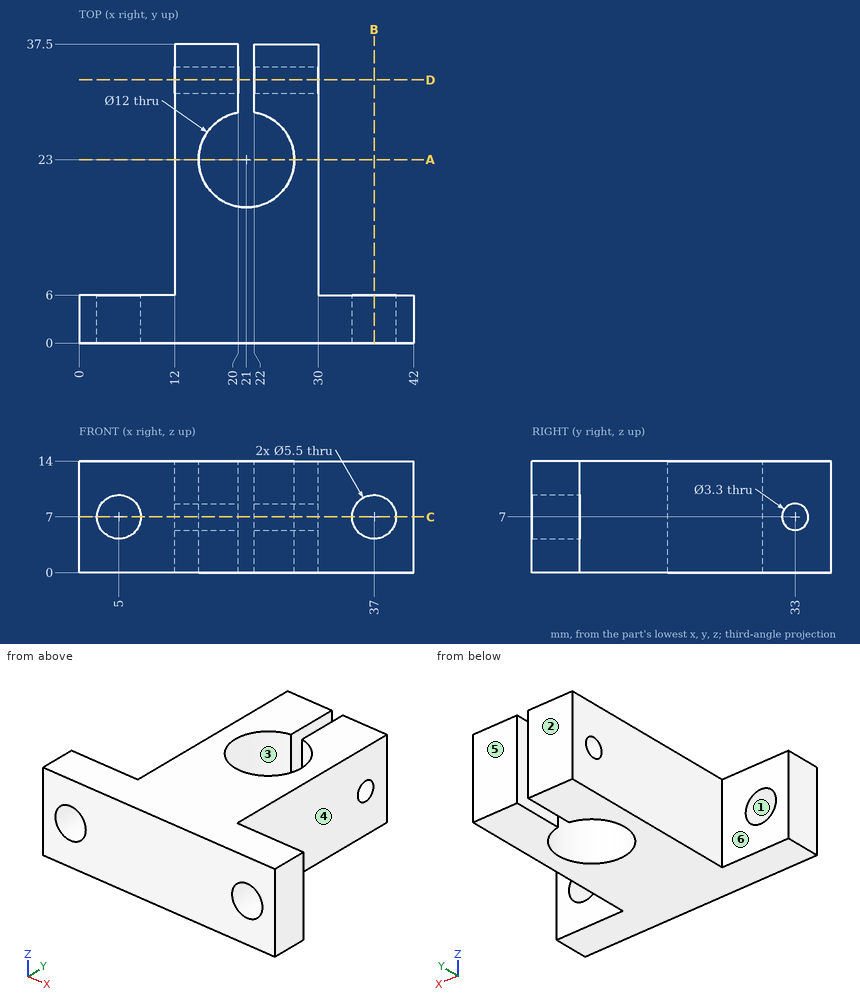
Study the drawing (mm; zero at the part's minimum x, y, z) and answer. A direction names the side the tool comes from. Give positions to 0.01 mm unless a question says otherwise; leave off trailing zeros. Write each loop counter-clockwise with the first axis right and the second up, starting at its lowest first coordinate (ties: lowest second). Pieces come first, ordered by that corner, then holes. Notation, with made-up numbers: (46.25, -31) - (62.25, -31) arc R35 ccw to (62.25, 5) - close; hole circle Ø11 at (29.25, -32). An arc over 180 degrees is marked (long way). Use a Markdown table: item, result.
1. A tool of negligible diameter and unlimited length cuts with its end or side. For the marked faces 4, 5 and 6, from which of +Z, -Z, +X, -X, +Y, -Y can it reach the whole face along a straight path? Write none if from no direction.
Values follow:
| item | result |
|---|---|
| face 4 | +Z, -Z, +X, +Y |
| face 5 | +Z, -Z, +X, -X, +Y |
| face 6 | +Z, -Z, -X, +Y |
2. Section D-D on y = 33 is taken. Write down the section's boundary in (x, z).
Values follow:
| item | result |
|---|---|
| outline | (12, 0) - (20, 0) - (20, 5.35) - (12, 5.35) - close; (12, 8.65) - (20, 8.65) - (20, 14) - (12, 14) - close; (22, 0) - (30, 0) - (30, 5.35) - (22, 5.35) - close; (22, 8.65) - (30, 8.65) - (30, 14) - (22, 14) - close |
3. Each of these flat-tipped pins is pushed along its axis until it touches: P1, Ø3, axis at y = 33, z = 7, coming from the -X side; P2, Ø4, axis at y = 23.5, z = 6, coming from the +X side; P3, Ø7, axis at y = 31.5, z = 10, coming from the -X side. Where does it stop, or does it pass through?
Values follow:
| item | result |
|---|---|
| P1 | passes through |
| P2 | stops at x = 30 |
| P3 | stops at x = 12 |
4. Section A-A on y = 23 is taken. Write down the section's boundary in (x, z), plus the area to 3 significant figures.
Values follow:
| item | result |
|---|---|
| outline | (12, 0) - (15, 0) - (15, 14) - (12, 14) - close; (27, 0) - (30, 0) - (30, 14) - (27, 14) - close |
| area | 84.0 mm² |
5. Find the intervals of material crossed by probe 1 along X at (y, z) = (2.5, 6.75); probe 2 along Y at (x, z) = (26.25, 7); probe 3 along X at (y, z) = (23, 7), in increasing order. Write a range as from..to.
Values follow:
| item | result |
|---|---|
| probe 1 | x = 0..2.26, 7.74..34.26, 39.74..42 |
| probe 2 | y = 0..20.1, 25.9..31.35, 34.65..37.5 |
| probe 3 | x = 12..15, 27..30 |
6. Section C-C on z = 7 is taken. Write down the section's boundary in (x, y).
Values follow:
| item | result |
|---|---|
| outline | (0, 0) - (2.25, 0) - (2.25, 6) - (0, 6) - close; (7.75, 0) - (34.25, 0) - (34.25, 6) - (30, 6) - (30, 31.35) - (22, 31.35) - (22, 28.92) arc R6 cw (long way) to (20, 28.92) - (20, 31.35) - (12, 31.35) - (12, 6) - (7.75, 6) - close; (12, 34.65) - (20, 34.65) - (20, 37.5) - (12, 37.5) - close; (22, 34.65) - (30, 34.65) - (30, 37.5) - (22, 37.5) - close; (39.75, 0) - (42, 0) - (42, 6) - (39.75, 6) - close |
7. Section B-B on x = 37 is taken. Write down the section's boundary in (y, z), plus the area to 3 significant figures.
Values follow:
| item | result |
|---|---|
| outline | (0, 0) - (6, 0) - (6, 4.25) - (0, 4.25) - close; (0, 9.75) - (6, 9.75) - (6, 14) - (0, 14) - close |
| area | 51.0 mm² |
8. For a pull along Y with two mould halves and no side action, classify the marked faces 1, 2 and 3 as released by +Y, released by -Y, zero draft, split by the parting line, or undercut.
Values follow:
| item | result |
|---|---|
| face 1 | zero draft |
| face 2 | released by +Y |
| face 3 | undercut |
